The drawing under review shows one solid part. Ordinate dimensions are in mm from its lowest x, y, z. Give positions to 0.01 mm unless a question says otherwise; leave off trailing zeros. Order: outer loops, then holes, each group sorted by start corner. A loop starts at its lowest first (then second) coordinate and runs counter-clockwise, first axis right, second up. Notation, with made-up numbers: M -29.5,-23.5 L -6.5,-23.5 A24 ccw -6.5,13.5 Z; hole C -14,-39.5 d6. An arc over 180 degrees is marked long. Put each result on its own line as item: value. Start each with the question number.
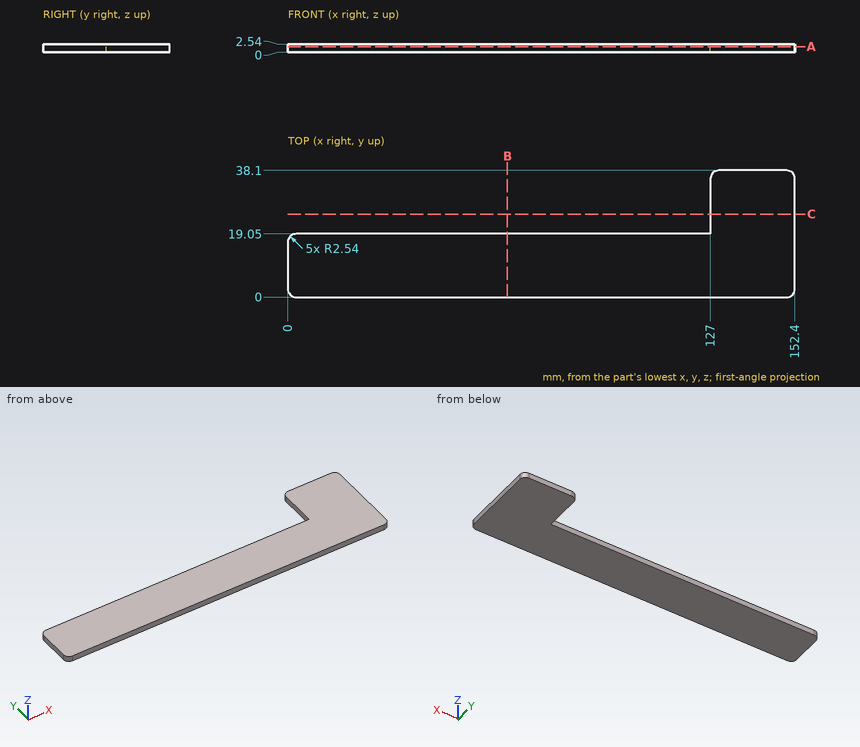
1. Consider section B-B on x = 66. Give the boundary of the cut face in (y, z).
2. Insertion check: pin 1 (1.3 mm diameter, centred on x = 74.5, z = 1, fed in from +Y); pin 2 (10 mm diameter, centred on x = 56, y = 27, fed in from +Z). Each pin has a flat end and moves straight along its axis. Give the tip position at first contact, or say it passes through.
3. Consider section A-A on z = 1.75. Give the boundary of the cut face in (x, y), then the cut area to 3 significant figures.
4. Consider section C-C on y = 25. Give the boundary of the cut face in (x, z).
5. To check wall thickness, follow probe 1 along X at (y, z) = (27.5, 1.4); probe 2 along Y at (x, z) = (77, 1.6); probe 3 along X at (y, z) = (36.5, 2.45). State the ranges of each line that lie inside material, in increasing order.
Returned:
1. outline: M 0,0 L 19.05,0 L 19.05,2.54 L 0,2.54 Z
2. pin 1: stops at y = 19.05
2. pin 2: passes through
3. outline: M 0,2.54 A2.54 ccw 2.54,0 L 149.86,0 A2.54 ccw 152.4,2.54 L 152.4,35.56 A2.54 ccw 149.86,38.1 L 129.54,38.1 A2.54 ccw 127,35.56 L 127,19.05 L 2.54,19.05 A2.54 ccw 0,16.51 Z
3. area: 3,380 mm2
4. outline: M 127,0 L 152.4,0 L 152.4,2.54 L 127,2.54 Z
5. probe 1: x = 127 to 152.4
5. probe 2: y = 0 to 19.05
5. probe 3: x = 127.18 to 152.22
